The model under review builds one solid part; all positions refer to its coordinate system, in mm. Face numbers are marked on the shaded views. A direction names the side the tool comes from. Round coordinates to 2 decimals unless told otherwise and drop trailing zeros. Loops run counter-clockwise (first coordinate to the right, second up) from the corner with the lowest first, then second, coordinate; pieces in that order, holes last. Notation, with made-up numbers: (-19.75, 24.25) -> (1.25, 24.25) arc R15 ccw to (1.25, 50.25) -> close; hole circle Ø8 at (57.5, 87). An arc over 180 degrees is marked (long way). Use a Markdown table: item, result. Add a question column.
1) Consider section C-C on y = -2.5. Give the boundary of the cut face in (x, z).
2) Wall thickness on probe 1 along Y at (x, z) = (3, -0.75); probe 2 along X at (y, z) = (6, -6.75); probe 3 along X at (y, z) = (0.75, 1.25): over which ranges is each line inside the solid? List them lowest first.
3) Insertion check: pin 1 (11.5 mm diameter, centred on x = 18, y = -1.5, fed in from -Z); pin 2 (10.5 mm diameter, centred on x = 0, y = 0, fed in from -Z); pin 3 (1.6 mm diameter, centred on x = 23, y = 12, fed in from +Z). Each pin has a flat end and moves straight along its axis. Give the tip position at first contact, or say it passes through.
4) Consider section A-A on x = 6. Give the boundary of the cut face in (y, z).
5) Consider section B-B on z = -2.5. State how many separate pieces and enclosed holes the cut face has, plus the area to 3 significant figures.
6) Mouldability with a two-part tool opening along Y and no side actions: class the marked faces 3, 4 and 5 as released by +Y, released by -Y, zero draft, split by the parting line, or undercut.
7) Consider section D-D on z = 1.25. Give the boundary of the cut face in (x, y).
8) For the marked faces 1 and 2, list the 3-axis set-ups (+Z, -Z, +X, -X, +Y, -Y) from which the entire face can be reached by the end or side of a thin tool; tool diameter is ignored.
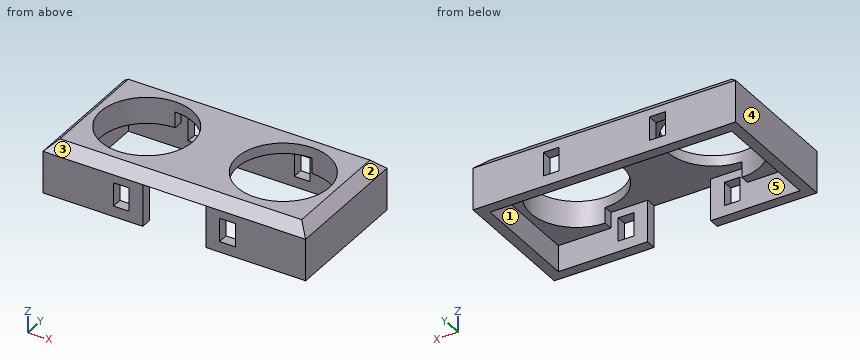
Autodesk Inventor part; units mm, degrees
ref_plane "YZ Plane" through (0, 0, 0) normal (1, 0, 0) x (0, 1, 0)
ref_plane "XZ Plane" through (0, 0, 0) normal (0, 1, 0) x (-1, 0, 0)
ref_plane "XY Plane" through (0, 0, 0) normal (0, 0, 1) x (1, 0, 0)
sketch "Sketch1" plane through (0, 0, 0) normal (0, 0, 1) x (1, 0, 0)
  circle A0 centre (0, 0) radius 8.75
  circle A1 centre (26, 0) radius 8.75
  line L0 (-12, 12.5) -> (38, 12.5)
  line L1 (38, 12.5) -> (38, -12.5)
  line L2 (38, -12.5) -> (-12, -12.5)
  line L3 (-12, -12.5) -> (-12, 12.5)
  dimension "d0" = 17.5
  dimension "d1" = 17.5
  dimension "d2" = 26
  dimension "d3" = 50
  dimension "d4" = 25
  dimension "d5" = 12
  dimension "d6" = 12.5
extrude "Extrusion1" add sketch "Sketch1" along normal blind 2
sketch "Sketch2" plane through (0, 0, 0) normal (0, 0, -1) x (-1, 0, 0)
  line L0 (-38, 12.5) -> (12, 12.5)
  line L1 (12, -12.5) -> (-38, -12.5)
  line L2 (-38, 12.5) -> (12, 12.5)
  line L3 (12, 12.5) -> (12, -12.5)
  line L4 (-38, -12.5) -> (-38, 12.5)
  line L5 (-36, 10.5) -> (10, 10.5)
  line L6 (10, 10.5) -> (10, -10.5)
  line L7 (-36, -10.5) -> (-36, 10.5)
  line L8 (-19, -10.5) -> (-19, -12.5)
  line L9 (-7, -10.5) -> (-7, -12.5)
  line L10 (10, -10.5) -> (-7, -10.5)
  line L11 (-19, -10.5) -> (-36, -10.5)
  line L12 (12, -12.5) -> (-7, -12.5)
  line L13 (-19, -12.5) -> (-38, -12.5)
  point P0 (0, 0)
  point P1 (12, 12.5)
  point P2 (-19, -12.5)
  point P3 (-7, -12.5)
  dimension "d12" = 2
  dimension "d14" = 46
  dimension "d16" = 21
  dimension "d19" = 12
  dimension "d20" = 19
  dimension "d21" = 2
  dimension "d22" = 2
  dimension "d23" = 25
extrude "Extrusion2" add sketch "Sketch2" along normal blind 8 contours L0 L3 L1 L9 L10 L6 L5 L7 L11 L8 L4
sketch "Sketch3" plane through (0, 0, 0) normal (0, 0, -1) x (-1, 0, 0)
  circle A0 centre (-26, 0) radius 8.75
  arc A1 (-26, 8.75) -> (-34.75, 0) centre (-26, 0) ccw
  line L0 (-36, 10.5) -> (-36, -10.5)
  line L1 (-36, 10.5) -> (-26, 10.5)
  line L2 (10, 10.5) -> (-36, 10.5)
  line L3 (-26, 8.75) -> (-26, 10.5)
  arc A2 (-34.75, 0) -> (-26, -8.75) centre (-26, 0) ccw
  line L4 (-26, -8.75) -> (-26, -10.5)
  line L5 (-19, -10.5) -> (-36, -10.5)
  line L6 (-36, -10.5) -> (-26, -10.5)
  line L7 (-36, 0) -> (-36, -10.5)
  circle A3 centre (0, 0) radius 8.75
  arc A4 (8.75, 0) -> (0, 8.75) centre (0, 0) ccw
  arc A5 (0, -8.75) -> (8.75, 0) centre (0, 0) ccw
  line L8 (0, -8.75) -> (0, -10.5)
  line L9 (0, -10.5) -> (10, -10.5)
  line L10 (10, -10.5) -> (10, 10.5)
  line L11 (0, 10.5) -> (0, 8.75)
  point P0 (-26, 9.625)
  point P1 (-35.375, 0)
  point P2 (-26, -9.625)
  point P3 (0, 9.625)
extrude "Extrusion3" add sketch "Sketch3" along normal blind 3 contours A0 L4 L5 L0 L1 L3 | L10 L9 L8 A3 L11 L2
chamfer "Chamfer2" distance 2 angle 45 4 edges at (13, 12.5, 2) (13, -12.5, 2) (38, 0, 2) (-12, 0, 2)
sketch "Sketch5" plane through (19, -12.5, -8) normal (0, -1, 0) x (1, 0, 0)
  line L0 (5.6, 2) -> (2.6, 2)
  line L1 (2.6, 2) -> (2.6, 6.5)
  line L2 (2.6, 6.5) -> (5.6, 6.5)
  line L3 (5.6, 6.5) -> (5.6, 2)
  line L4 (-14.6, 2) -> (-17.6, 2)
  line L5 (-17.6, 2) -> (-17.6, 6.5)
  line L6 (-17.6, 6.5) -> (-14.6, 6.5)
  line L7 (-14.6, 6.5) -> (-14.6, 2)
  line L8 (19, 0) -> (19, 10)
  line L9 (0, 8) -> (19, 8)
  line L10 (19, 0) -> (0, 0)
  line L11 (-31, 8) -> (-12, 8)
  point P0 (-19, 8)
  dimension "d29" = 3
  dimension "d31" = 3
  dimension "d33" = 17.2
  dimension "d34" = 13.4
  dimension "d35" = 1.5
  dimension "d38" = 2
  dimension "d39" = 1.5
extrude "Extrusion4" cut sketch "Sketch5" against normal through all
properties part number "UltrasonicSensorMountTest"
Result set:
| question | item | result |
|---|---|---|
| 1 | outline | (-12, -8) -> (-10, -8) -> (-10, -3) -> (-8.39, -3) -> (-8.39, 2) -> (-10, 2) -> (-12, 0) -> close; (8.39, 0) -> (17.61, 0) -> (17.61, 2) -> (8.39, 2) -> close; (34.39, -3) -> (36, -3) -> (36, -8) -> (38, -8) -> (38, 0) -> (36, 2) -> (34.39, 2) -> close |
| 2 | probe 1 | -12.5 to -10.5, 10.5 to 12.5 |
| 2 | probe 2 | -12 to -10, 36 to 38 |
| 2 | probe 3 | -10.75 to -8.72, 8.72 to 17.28, 34.72 to 36.75 |
| 3 | pin 1 | z = 0 |
| 3 | pin 2 | through |
| 3 | pin 3 | z = 1.3 |
| 4 | outline | (-12.5, -8) -> (-10.5, -8) -> (-10.5, 0) -> (-6.37, 0) -> (-6.37, 2) -> (-10.5, 2) -> (-12.5, 0) -> close; (6.37, 0) -> (10.5, 0) -> (10.5, -8) -> (12.5, -8) -> (12.5, 0) -> (10.5, 2) -> (6.37, 2) -> close |
| 5 | separate pieces | 5 |
| 5 | enclosed holes | 0 |
| 5 | area | 415 mm2 |
| 6 | face 3 | released by -Y |
| 6 | face 4 | zero draft |
| 6 | face 5 | undercut |
| 7 | outline | (-10.75, -11.25) -> (36.75, -11.25) -> (36.75, 11.25) -> (-10.75, 11.25) -> close; hole circle Ø17.5 at (0, 0); hole circle Ø17.5 at (26, 0) |
| 8 | face 1 | -Z |
| 8 | face 2 | +Z, +X, +Y, -Y |
